Verification items for the finished model (mm, model axes). A direction names the side the tool comes from. Coordinates: 2 decimals unless noted, no trailing zeros. Loops run counter-clockwise (first coordinate to the right, second up) from the corner with the lowest first, then second, coordinate; pieces in that order, holes last. Notation, with made-up numbers: (88.5, 74) - (100.5, 74) arc R28 ccw to (100.5, 96) - close; hole circle Ø11 at (-31.75, 71). An arc over 180 degrees is marked (long way). One line per item, written item: value. Start each with the question number.
(1) Thickness scan on probe 1 along Y at (x, z) = (-27.5, 5.5); probe 2 along Y at (x, z) = (18, 14.75); probe 3 along X at (y, z) = (29.5, 16.75). Record the ranges inside material, lowest first. Write a range as [from, to].
(2) Gauge pin test, flat ends, axial feed: P1, Ø4, axis at y = 47.5, z = 11, coming from the +X side; P2, Ø1, axis at y = 8.5, z = 15.5, coming from the +X side; P3, Ø1, axis at x = -18.5, z = 8.5, coming from the -Y side; P4, Ø2, axis at x = -18, y = 22, coming from the -Z side. Record the tip position at first contact, or that the pin passes through.
(3) Section check B-B (y = 9.5). Record the boundary of the cut face in (x, z).
(4) Set-up check for faces 4 (the face through (-20.167, -5.07, 9.86)), 5 (the face through (39, 14.5, 10)), 6 (the face through (-29.734, 36.535, 9.785)), 7 (the face through (23, 19.5, 10)), 8 (the face through (36, 39, 10)): record each of +Z, -Z, +X, -X, +Y, -Y from which the full face is reachable in a straight line by a thin tool's end or side.
(5) Draft check along X on faces 1 (the face through (-7.6, 24, 10)), 2 (the face through (-12.8, 44.83, 9.86)), 3 (the face through (12.89, 44.67, 9.86)). Enter one of: +X half, -X half, draft (parallel to the pull), parting line (faces both ways), or undercut.
(6) Section check C-C (x = 43). Record the boundary of the cut face in (y, z).
(7) Section check D-D (z = 10). Count the separate pieces of the cut face and the enclosed holes in it, plus the area to 3 significant figures.
(8) Section check A-A (x = 0). Record the boundary of the cut face in (y, z).
```python
from build123d import *

# Parameters (mm, degrees)
SKETCH_1_R          = 1.65
SKETCH_1_R_2        = 5
EXTRUDE_1_DEPTH     = 20
SKETCH_2_R          = 1.65
CUT_EXTRUDE_1_DEPTH = 71.32780389
EXTRUDE_START       = -20
EXTRUDE_2_DEPTH     = 20
SKETCH_4_R          = 1.65
CUT_EXTRUDE_2_DEPTH = 82
EXTRUDE_5_DEPTH     = 20
CUT_EXTRUDE_3_DEPTH = 20
SKETCH_8_W          = 31.905989232
SKETCH_8_H          = 14.5
CUT_EXTRUDE_5_DEPTH = 82
CUT_EXTRUDE_6_DEPTH = 82
FILLET_3_R          = 1


with BuildPart() as part:
    # Sketch 1 → Extrude 1 (new body)
    with BuildSketch(Plane.XY):
        with BuildLine():
            Line((55, 39), (16.165807537, 39))
            Line((16.165807537, 39), (9.526279442, 50.5))
            ThreePointArc((9.526279442, 50.5), (0, 56), (-9.526279442, 50.5))
            Line((-9.526279442, 50.5), (-16.165807537, 39))
            Line((-16.165807537, 39), (-55, 39))
            Line((-55, 39), (-55, 0))
            Line((-55, 0), (-14.1, 0))
            ThreePointArc((-14.1, 0), (0, 14.1), (14.1, 0))
            Line((14.1, 0), (55, 0))
            Line((55, 0), (55, 39))
        make_face()
        with Locations((-8, 45)):
            Circle(SKETCH_1_R, mode=Mode.SUBTRACT)
        with Locations((0, 45)):
            Circle(SKETCH_1_R_2, mode=Mode.SUBTRACT)
        with Locations((8, 45)):
            Circle(SKETCH_1_R, mode=Mode.SUBTRACT)
        with Locations((0, 53)):
            Circle(SKETCH_1_R, mode=Mode.SUBTRACT)
    extrude(amount=EXTRUDE_1_DEPTH)

    # Sketch 2 → Cut-Extrude 1 (cut, through all)
    with BuildSketch(Plane(origin=(0, 39, 0), x_dir=(1, 0, 0), z_dir=(0, 1, 0))):
        with Locations(Location((-50, -10, 0), (0, 0, 270))):
            Circle(SKETCH_2_R)
        with Locations(Location((-31.37, -10, 0), (0, 0, 270))):
            Circle(SKETCH_2_R)
        with Locations(Location((31.37, -10, 0), (0, 0, 270))):
            Circle(SKETCH_2_R)
        with Locations(Location((50, -10, 0), (0, 0, 270))):
            Circle(SKETCH_2_R)
    extrude(amount=-CUT_EXTRUDE_1_DEPTH, mode=Mode.SUBTRACT)

    # Sketch 3 → Extrude 2 (add)
    with BuildSketch(Plane.XY.offset(20).offset(EXTRUDE_START)):
        with BuildLine():
            ThreePointArc((-20, 0), (-19.318516526, -5.176380902), (-17.320508076, -10))
            Line((-17.320508076, -10), (-9.940321926, -10))
            ThreePointArc((-9.940321926, -10), (-13.018612429, -5.415323667), (-14.1, 0))
            Line((-14.1, 0), (-20, 0))
        make_face()
        with BuildLine():
            Line((9.940321926, -10), (17.320508076, -10))
            ThreePointArc((17.320508076, -10), (19.318516526, -5.176380902), (20, 0))
            Line((20, 0), (14.1, 0))
            ThreePointArc((14.1, 0), (13.018612429, -5.415323667), (9.940321926, -10))
        make_face()
    extrude(amount=EXTRUDE_2_DEPTH)

    # Sketch 4 → Cut-Extrude 2 (cut, through all)
    with BuildSketch(Plane.XY.offset(20)):
        with Locations((17, 0)):
            Circle(SKETCH_4_R)
        with Locations((-17, 0)):
            Circle(SKETCH_4_R)
    extrude(amount=-CUT_EXTRUDE_2_DEPTH, mode=Mode.SUBTRACT)

    # Sketch 5 → Extrude 5 (add)
    with BuildSketch(Plane.XY.offset(20).offset(EXTRUDE_START)):
        with BuildLine():
            Line((-17.320508076, -10), (-23.094010768, 0))
            Line((-23.094010768, 0), (-20, 0))
            ThreePointArc((-20, 0), (-19.318516526, -5.176380902), (-17.320508076, -10))
        make_face()
        with BuildLine():
            Line((17.320508076, -10), (23.094010768, 0))
            Line((23.094010768, 0), (20, 0))
            ThreePointArc((20, 0), (19.318516526, -5.176380902), (17.320508076, -10))
        make_face()
    extrude(amount=EXTRUDE_5_DEPTH)

    # Sketch 6 → Cut-Extrude 3 (cut)
    with BuildSketch(Plane.XY.offset(20)):
        with BuildLine():
            Line((3.806573262, 31.6), (-3.806573262, 31.6))
            ThreePointArc((-3.806573262, 31.6), (-6.01040764, 30.01040764), (-7.6, 27.806573262))
            Line((-7.6, 27.806573262), (-7.6, 20.193426738))
            ThreePointArc((-7.6, 20.193426738), (-6.01040764, 17.98959236), (-3.806573262, 16.4))
            Line((-3.806573262, 16.4), (3.806573262, 16.4))
            ThreePointArc((3.806573262, 16.4), (6.01040764, 17.98959236), (7.6, 20.193426738))
            Line((7.6, 20.193426738), (7.6, 27.806573262))
            ThreePointArc((7.6, 27.806573262), (6.01040764, 30.01040764), (3.806573262, 31.6))
        make_face()
    extrude(amount=-CUT_EXTRUDE_3_DEPTH, mode=Mode.SUBTRACT)

    # Sketch 8 → Cut-Extrude 5 (cut, through all)
    with BuildSketch(Plane(origin=(0, 0, 0), x_dir=(-1, 0, 0), z_dir=(0, 0, -1))):
        with Locations((-39.047005384, 7.25)):
            Rectangle(SKETCH_8_W, SKETCH_8_H)
        with Locations((39.047005384, 7.25)):
            Rectangle(SKETCH_8_W, SKETCH_8_H)
    extrude(amount=-CUT_EXTRUDE_5_DEPTH, mode=Mode.SUBTRACT)

    # Sketch 9 → Cut-Extrude 6 (cut, through all)
    with BuildSketch(Plane(origin=(0, 0, 0), x_dir=(-1, 0, 0), z_dir=(0, 0, -1))):
        Polygon((-47, 34), (-47, 19.5), (-22.435993944, 34), align=None)
        Polygon((-37.164006056, 19.5), (-12.6, 34), (-12.6, 19.5), align=None)
        Polygon((12.6, 19.5), (37.164006056, 19.5), (12.6, 34), align=None)
        Polygon((22.435993944, 34), (47, 34), (47, 19.5), align=None)
    extrude(amount=-CUT_EXTRUDE_6_DEPTH, mode=Mode.SUBTRACT)

    # Fillet 3
    fillet_3_edges = [part.edges().sort_by_distance(p)[0] for p in [
        (12.6, 19.5, 10),
        (37.164006056, 19.5, 10),
        (12.6, 34, 10),
        (-12.6, 34, 10),
        (-37.164006056, 19.5, 10),
        (-12.6, 19.5, 10),
        (-47, 19.5, 10),
        (-22.435993944, 34, 10),
        (-47, 34, 10),
        (47, 34, 10),
        (22.435993944, 34, 10),
        (47, 19.5, 10),
    ]]
    fillet(fillet_3_edges, radius=FILLET_3_R)


solid = part.part
```
Responses:
1. probe 1: y = [14.5, 19.5], [25.2, 31.01], [34, 39]
1. probe 2: y = [-8.82, -1.31], [1.31, 19.5], [30.81, 39]
1. probe 3: x = [-55, -47], [-30.06, -20.22], [-12.6, -6.48], [6.48, 12.6], [20.22, 30.06], [47, 55]
2. P1: stops at x = 12.41
2. P2: stops at x = 23.09
2. P3: stops at y = -8.82
2. P4: passes through
3. outline: (-23.09, 0) - (-10.42, 0) - (-10.42, 20) - (-23.09, 20) - close; (10.42, 0) - (23.09, 0) - (23.09, 20) - (10.42, 20) - close
4. face 4: +Z, -Z, -X, -Y
4. face 5: +Z, -Z, +X, -Y
4. face 6: +Y, -Y
4. face 7: +Z, -Z
4. face 8: +Z, -Z, +X, +Y
5. face 1: undercut
5. face 2: -X half
5. face 3: +X half
6. outline: (14.5, 0) - (21.86, 0) - (21.86, 20) - (14.5, 20) - close; (34, 0) - (39, 0) - (39, 20) - (34, 20) - close
7. separate pieces: 5
7. enclosed holes: 7
7. area: 2,280 mm²
8. outline: (14.1, 0) - (16.4, 0) - (16.4, 20) - (14.1, 20) - close; (31.6, 0) - (40, 0) - (40, 20) - (31.6, 20) - close; (50, 0) - (51.35, 0) - (51.35, 20) - (50, 20) - close; (54.65, 0) - (56, 0) - (56, 20) - (54.65, 20) - close
